The figure shows three views and two pictorial views of one solid part (mm, origin at its lowest corner). Answer the questions. A direction names the side the tool comes from. Round coordinates to 2 decimals unless told otherwise and drop trailing zeros. Loops run counter-clockwise (first coordinate to the right, second up) from the corner with the lowest first, then second, coordinate; pieces in that order, holes last. Notation, with made-up numbers: (-24.5, -29) -> (-0.5, -29) arc R18 ccw to (-0.5, -17) -> close; hole circle Ø1 at (-13.75, 70). An arc over 180 degrees is marked (long way). Write item = value, one per line. Start each with the question number.
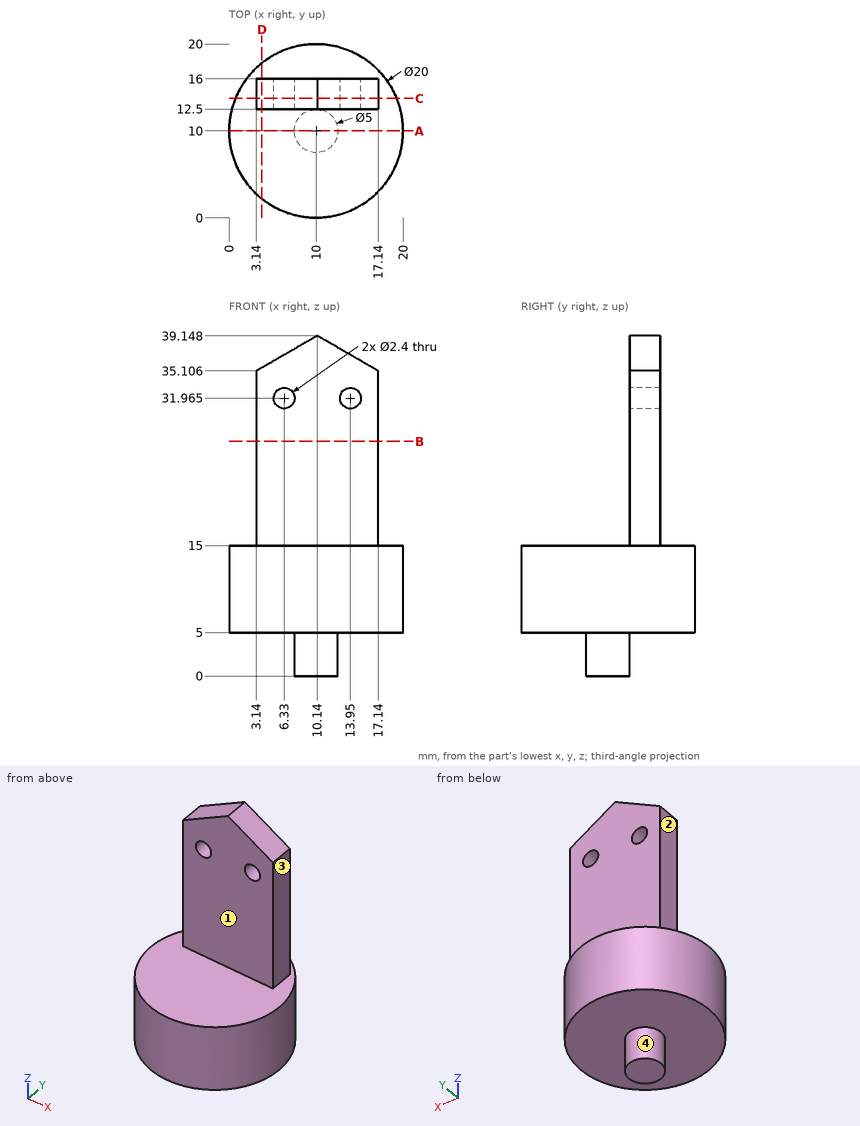
Item 1: A tool of negligible diameter and unlimited length cuts with its end or side. For the marked faces 1, 2, 3 and 4, from which of +Z, -Z, +X, -X, +Y, -Y can it reach the whole face along a straight path? Write none if from no direction.
Item 2: Section C-C (y = 13.75) is taken. Count the separate pieces of the cut face and the enclosed holes in it, then the cut area to 3 significant figures.
Item 3: Section A-A (y = 10) is taken. Determine the outline of the cut face in (x, z).
Item 4: Section D-D (x = 3.75) is taken. Determine the outline of the cut face in (y, z).
Item 5: Flat-ended cylindrical pins translate along their axes: pin 1 (1.5 mm diameter, centred on x = 6.5, y = 10.5, fed in from +Z); pin 2 (2 mm diameter, centred on x = 3.5, y = 12, fed in from -Z); pin 3 (7 mm diameter, centred on x = 10, z = 21.5, fed in from +Y). Find the tip coordinate at first contact, or state that the pin passes through.
Item 6: Find the intervals of material crossed by line 1 along Y through (x, z) = (14.5, 34.5); line 2 along Z through (x, y) = (14.5, 3.25); line 3 along Z through (x, y) = (9.5, 7.75), in increasing order. Write a range as [from, to].
Item 7: Section B-B (z = 27) is taken. Determine the outline of the cut face in (x, y).
Worked answers:
q1.face_1 = +Z, +X, -X, -Y
q1.face_2 = +Z, -X, +Y, -Y
q1.face_3 = +Z, +X, +Y, -Y
q1.face_4 = -Z
q2.separate_pieces = 1
q2.enclosed_holes = 2
q2.area = 486 mm2
q3.outline = (0, 5) -> (7.5, 5) -> (7.5, 0) -> (12.5, 0) -> (12.5, 5) -> (20, 5) -> (20, 15) -> (0, 15) -> close
q4.outline = (2.19, 5) -> (17.81, 5) -> (17.81, 15) -> (16, 15) -> (16, 35.46) -> (12.5, 35.46) -> (12.5, 15) -> (2.19, 15) -> close
q5.pin_1 = 15
q5.pin_2 = 5
q5.pin_3 = 16
q6.line_1 = [12.5, 16]
q6.line_2 = [5, 15]
q6.line_3 = [0, 15]
q7.outline = (3.14, 12.5) -> (17.14, 12.5) -> (17.14, 16) -> (3.14, 16) -> close
